Geometry: final body of the model. Coordinates: model frame, mm. Face numbers are marked on the shaded views. A direction names the side the tool comes from. Give positions to 0.01 mm unless a question says otherwise; leave off trailing zeros. Write each loop counter-clockwise with the first axis right and the second up, starting at its lowest first coordinate (ties: lowest second). Pieces come first, ordered by that corner, then holes. Notation, with made-up numbers: (18.25, 35.5) - (62.25, 35.5) arc R33 cw to (62.25, 63.5) - close; hole circle Ø3 at (-32, 1.25). An arc over 180 degrees is marked (long way). Use CSV: the item, a comma, the result in double quotes. Start each with the question number.
(1) Reachability of the marked faces 1, 2, 3, 4 and 5 from +Z, -Z, +X, -X, +Y, -Y: full face, straight path, thin tool, end or side. Return the list, or none.
(2) Section B-B on x = 20.5. Output: boundary loops of the cut face in (y, z), and give its area (3 significant figures).
(3) Section C-C on z = 20. Output: boundary loops of the cut face in (x, y), and give its area (3 significant figures).
(4) Section A-A on y = -14. Output: boundary loops of the cut face in (x, z), and give its area (3 significant figures).
(5) Draft query along Y for the marked faces 6, 7 and 8. Return one class per face: released by +Y, released by -Y, zero draft, split by the parting line, or undercut.
(6) First-contact query: pin 1 Ø4 at (x, y) = (9, -10) entering from +Z; pin 2 Ø8 at (y, z) = (-52, -15) entering from -X; pin 3 Ø10 at (x, y) = (12.5, -23) entering from -Z. Flat tips, straight axial feed; report the tip coordinate or a pass-through.
(7) Section D-D on x = -9.5. Output: boundary loops of the cut face in (y, z).
(8) Line query: probe 1 along X at (y, z) = (3, 0); probe 2 along X at (y, z) = (-46.5, -8); probe 3 along Y at (x, z) = (23, -10). Output: solid intervals per line, ascending. Write a range as [from, to].
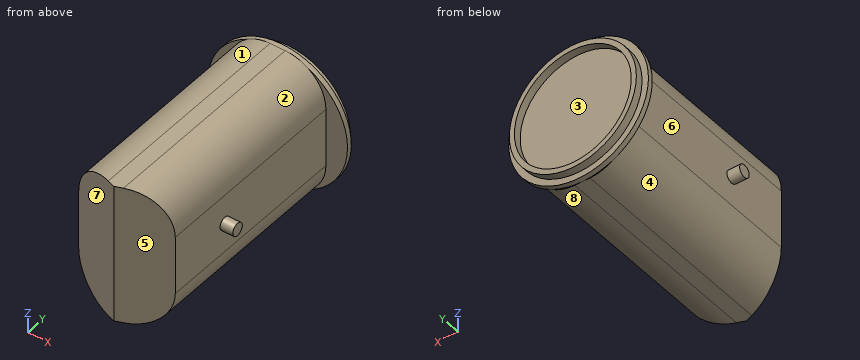
from build123d import *

# Parameters (mm, degrees)
SKETCH1_R           = 27.5
BOSS_EXTRUDE1_DEPTH = 2
SKETCH2_R           = 25
SKETCH2_R_2         = 23
BOSS_EXTRUDE2_DEPTH = 3
BOSS_EXTRUDE3_DEPTH = 87
CHAMFER2_SIZE       = 8
CHAMFER2_SIZE_2     = 21.979819356
SKETCH5_R           = 2.5
BOSS_EXTRUDE4_DEPTH = 5


with BuildPart() as part:
    # Sketch1 → Boss-Extrude1 (new body)
    with BuildSketch(Plane(origin=(0, 0, 0), x_dir=(1, 0, 0), z_dir=(0, 1, 0))):
        with Locations(Location((0, 0, 0), (0, 0, 270))):
            Circle(SKETCH1_R)
    extrude(amount=BOSS_EXTRUDE1_DEPTH)

    # Sketch2 → Boss-Extrude2 (add)
    with BuildSketch(Plane(origin=(0, 2, 0), x_dir=(1, 0, 0), z_dir=(0, 1, 0))):
        with Locations(Location((0, 0, 0), (0, 0, 270))):
            Circle(SKETCH2_R)
        with Locations(Location((0, 0, 0), (0, 0, 270))):
            Circle(SKETCH2_R_2, mode=Mode.SUBTRACT)
    extrude(amount=BOSS_EXTRUDE2_DEPTH)

    # Sketch3 → Boss-Extrude3 (add)
    with BuildSketch(Plane.XZ):
        with BuildLine():
            Line((3, -27.5), (-3, -27.5))
            ThreePointArc((-3, -27.5), (-14.313708499, -22.813708499), (-19, -11.5))
            Line((-19, -11.5), (-19, 11.5))
            ThreePointArc((-19, 11.5), (-14.313708499, 22.813708499), (-3, 27.5))
            Line((-3, 27.5), (3, 27.5))
            ThreePointArc((3, 27.5), (14.313708499, 22.813708499), (19, 11.5))
            Line((19, 11.5), (19, -11.5))
            ThreePointArc((19, -11.5), (14.313708499, -22.813708499), (3, -27.5))
        make_face()
    extrude(amount=BOSS_EXTRUDE3_DEPTH)

    # Chamfer2
    # the kernel refuses this chamfer: 21.979819356, 8 mm, written as the material it takes off along each edge
    with BuildSketch(Plane(origin=(19, -87, 68.519931595), x_dir=(0.0990409022520504, 0.9950833631817486, 0), z_dir=(0, 0, -1)), Plane(origin=(-19, -87, -68.519931595), x_dir=(-0.0990409022520504, 0.9950833631817486, 0), z_dir=(0, 0, 1))) as chamfer2_piece_1:
        Polygon((CHAMFER2_SIZE * 0.995083363182, -CHAMFER2_SIZE * 0.0990409022521), (-CHAMFER2_SIZE_2 * 0.0990409022504, -CHAMFER2_SIZE_2 * 0.995083363165), (0, 0), align=None)
    extrude(amount=137.03986319, mode=Mode.SUBTRACT)

    # Sketch5 → Boss-Extrude4 (add)
    with BuildSketch(Plane.ZY.offset(19)):
        with Locations(Location((0, -53, 0), (0, 0, 180))):
            Circle(SKETCH5_R)
    boss_extrude4 = extrude(amount=BOSS_EXTRUDE4_DEPTH)

    # Mirror1: Boss-Extrude4 across plane
    add(boss_extrude4.mirror(Plane(origin=(0, 0, 0), x_dir=(0, 0, 1), z_dir=(1, 0, 0))))


solid = part.part
Check values:
1,face 1,"+Z, -X, -Y"
1,face 2,"+Z, +X, -Y"
1,face 3,"+Y"
1,face 4,"-Z, -X, -Y"
1,face 5,"+Z, -Z, +X, -Y"
2,outline,"circle Ø5 at (-53, 0); (0, -18.33) - (2, -18.33) - (2, -14.31) - (5, -14.31) - (5, -10.43) - (2, -10.43) - (2, 10.43) - (5, 10.43) - (5, 14.31) - (2, 14.31) - (2, 18.33) - (0, 18.33) - close"
2,area,"116 mm²"
3,outline,"(-18.87, 0) - (-16.56, 0) - (-16.56, -79.89) - (0, -85.92) - (16.56, -79.89) - (16.56, 0) - (18.87, 0) - (18.87, 2) - (15, 2) - (15, 5) - (11.36, 5) - (11.36, 2) - (-11.36, 2) - (-11.36, 5) - (-15, 5) - (-15, 2) - (-18.87, 2) - close"
3,area,"2,840 mm²"
4,outline,"(-19, -11.5) arc R16 ccw to (-3, -27.5) - (3, -27.5) arc R16 ccw to (19, -11.5) - (19, 11.5) arc R16 ccw to (3, 27.5) - (-3, 27.5) arc R16 ccw to (-19, 11.5) - close"
4,area,"1,870 mm²"
5,face 6,"undercut"
5,face 7,"released by -Y"
5,face 8,"zero draft"
6,pin 1,"stops at z = 26.99"
6,pin 2,"stops at x = -19"
6,pin 3,"stops at z = -26.85"
7,outline,"(-82.46, -26.12) - (0, -26.12) - (0, -25.81) - (2, -25.81) - (2, -23.12) - (5, -23.12) - (5, -20.95) - (2, -20.95) - (2, 20.95) - (5, 20.95) - (5, 23.12) - (2, 23.12) - (2, 25.81) - (0, 25.81) - (0, 26.12) - (-82.46, 26.12) - close"
8,probe 1,"x = [-25, -23], [23, 25]"
8,probe 2,"x = [-19, 19]"
8,probe 3,"y = [0, 2]"
